from build123d import *

# Parameters (mm, degrees)
F1_DEPTH = 20


with BuildPart() as f1:
    # F0 (on Right) → F1 (new body)
    with BuildSketch(Plane.YZ):
        with BuildLine():
            Line((-30.74899, 39.781864), (-48.74899, 39.781864))
            ThreePointArc((-48.74899, 39.781864), (-52.284524, 38.317398), (-53.74899, 34.781864))
            Line((-53.74899, 34.781864), (-53.74899, -55.218136))
            ThreePointArc((-53.74899, -55.218136), (-52.284524, -58.75367), (-48.74899, -60.218136))
            Line((-48.74899, -60.218136), (38.41838, -60.218136))
            ThreePointArc((38.41838, -60.218136), (41.953914, -58.75367), (43.41838, -55.218136))
            Line((43.41838, -55.218136), (43.41838, -50.218136))
            ThreePointArc((43.41838, -50.218136), (41.953914, -46.682602), (38.41838, -45.218136))
            Line((38.41838, -45.218136), (-20.74899, -45.218136))
            ThreePointArc((-20.74899, -45.218136), (-24.284524, -43.75367), (-25.74899, -40.218136))
            Line((-25.74899, -40.218136), (-25.74899, 34.781864))
            ThreePointArc((-25.74899, 34.781864), (-27.213456, 38.317398), (-30.74899, 39.781864))
        make_face()
    extrude(amount=F1_DEPTH)


solid = f1.part
Could you check a few things on this model? Use its own coordinates, in mm. A direction names the side the tool comes from. Coordinates: 2 decimals unless noted, no trailing zeros. Order: outer loops, then holes, each group sorted by start corner. A loop starts at its lowest first (then second) coordinate and runs counter-clockwise, first axis right, second up. Notation, with made-up numbers: (69.5, 47) - (81.5, 47) arc R13 ccw to (81.5, 51) - close; hole circle Ø7 at (58, 37.5). An arc over 180 degrees is marked (long way). Answer in a Markdown table with one row per item. Add a question column.
(1) If we section it at A-A, the plane x = 4: Please give me the cut outline in (y, z), then the cut area to 3 significant figures.
(2) If we section it at B-B, the plane z = -3.5: Please give me the cut outline in (x, y).
(3) I need wall thicknesses on L1, parallel to Z at x = 1.5, y = 31.5; L2, parallel to Y at x = 7.5, z = 1. Which ranges of each line are inside material? Lowest first, please.
(4) On a 3-axis mill with a long thin cutter (end or side, diameter ignored), from which of +Z, -Z, +X, -X, +Y, -Y can I reach the whole of each face in a straight line? I mean faces 1 (the face through (10, 9, -45.218)), 2 (the face through (0, -27, -21)). Say none if no direction works.
(5) If we section it at C-C, the plane y = 25: Please give me the cut outline in (x, z).
(6) Will these pins go through, and if not, where does the flat tip stop? pin 1 (1.5 mm diameter, centred on x = 6.5, z = -47, fed in from +Y); pin 2 (6 mm diameter, centred on x = 11.5, y = 23.5, fed in from +Z).
Results are:
| question | item | result |
|---|---|---|
| 1 | outline | (-53.75, -55.22) arc R5 ccw to (-48.75, -60.22) - (38.42, -60.22) arc R5 ccw to (43.42, -55.22) - (43.42, -50.22) arc R5 ccw to (38.42, -45.22) - (-20.75, -45.22) arc R5 cw to (-25.75, -40.22) - (-25.75, 34.78) arc R5 ccw to (-30.75, 39.78) - (-48.75, 39.78) arc R5 ccw to (-53.75, 34.78) - close |
| 1 | area | 3,820 mm2 |
| 2 | outline | (0, -53.75) - (20, -53.75) - (20, -25.75) - (0, -25.75) - close |
| 3 | L1 | z = -60.22 to -45.22 |
| 3 | L2 | y = -53.75 to -25.75 |
| 4 | face 1 | +Z, +X, -X, +Y |
| 4 | face 2 | +Z, -Z, -X, +Y, -Y |
| 5 | outline | (0, -60.22) - (20, -60.22) - (20, -45.22) - (0, -45.22) - close |
| 6 | pin 1 | stops at y = 42.77 |
| 6 | pin 2 | stops at z = -45.22 |
